The listing builds one solid part. Answer for the finished solid, in the listing's coordinates (mm). Round coordinates to 2 decimals unless told otherwise and drop trailing zeros. Loops run counter-clockwise (first coordinate to the right, second up) from the corner with the lowest first, then second, coordinate; pieces in that order, holes last. Notation, with made-up numbers: (5, 56) - (15, 56) arc R22 cw to (15, 72) - close; hole circle Ø11 at (77, 31.5). An arc over 180 degrees is marked (long way). One line per item, written item: value.
```python
from build123d import *

# Parameters (mm, degrees)
BOSS_EXTRUDE1_DEPTH = 1.7272


with BuildPart() as part:
    # Sketch1 → Boss-Extrude1 (new body)
    with BuildSketch(Plane.XY):
        Polygon((-114.3, 13.37945), (-112.776, 13.37945), (-112.776, 15.10665), (-110.236, 15.10665), (-110.236, 13.37945), (-1.27, 13.37945), (-1.27, 15.10665), (1.27, 15.10665), (1.27, 13.37945), (110.236, 13.37945), (110.236, 15.10665), (112.776, 15.10665), (112.776, 13.37945), (114.3, 13.37945), (114.3, 12.61745), (116.0272, 12.61745), (116.0272, 10.58545), (114.3, 10.58545), (114.3, -7.70255), (116.0272, -7.70255), (116.0272, -9.73455), (114.3, -9.73455), (114.3, -13.37945), (112.776, -13.37945), (112.776, -15.10665), (110.236, -15.10665), (110.236, -13.37945), (1.27, -13.37945), (1.27, -15.10665), (-1.27, -15.10665), (-1.27, -13.37945), (-110.236, -13.37945), (-110.236, -15.10665), (-112.776, -15.10665), (-112.776, -13.37945), (-114.3, -13.37945), (-114.3, -9.73455), (-116.0272, -9.73455), (-116.0272, -7.70255), (-114.3, -7.70255), (-114.3, 10.58545), (-116.0272, 10.58545), (-116.0272, 12.61745), (-114.3, 12.61745), align=None)
        Polygon((-1.27, -1.517324769), (-72.54, -8.677584102), (-72.54, -9.56945), (-1.27, -9.56945), align=None, mode=Mode.SUBTRACT)
        Polygon((-78.89, -6.76276081), (-109.22, -9.80991481), (-109.22, 9.80991481), (-78.89, 6.76276081), align=None, mode=Mode.SUBTRACT)
        Polygon((-11.576521468, 0), (-72.54, -6.124797477), (-72.54, 6.124797477), align=None, mode=Mode.SUBTRACT)
        Polygon((-1.27, 9.56945), (-72.54, 9.56945), (-72.54, 8.677584102), (-1.27, 1.517324769), align=None, mode=Mode.SUBTRACT)
        Polygon((1.27, 1.517324769), (72.54, 8.677584102), (72.54, 9.56945), (1.27, 9.56945), align=None, mode=Mode.SUBTRACT)
        Polygon((78.89, 6.76276081), (109.22, 9.80991481), (109.22, -9.80991481), (78.89, -6.76276081), align=None, mode=Mode.SUBTRACT)
        Polygon((72.54, -6.124797477), (72.54, 6.124797477), (11.576521468, 0), align=None, mode=Mode.SUBTRACT)
        Polygon((1.27, -9.56945), (72.54, -9.56945), (72.54, -8.677584102), (1.27, -1.517324769), align=None, mode=Mode.SUBTRACT)
    extrude(amount=BOSS_EXTRUDE1_DEPTH)


solid = part.part
```
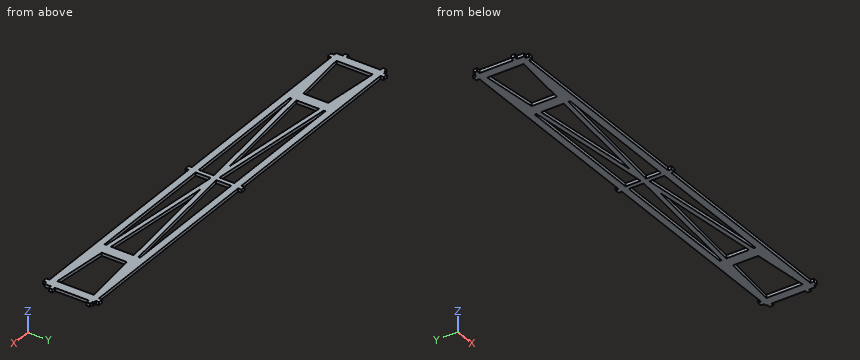
1) A cutting plane is placed at D-D on z = 0.45. Give the number of separate pieces and of enclosed holes in the cut face, and give its area (3 significant figures).
Final values:
separate pieces: 1
enclosed holes: 8
area: 3,130 mm2
2) A cutting plane is placed at C-C on x = -84.5. Give the vertices of the cut face in (y, z).
Final values:
outline: (-13.38, 0) - (-7.33, 0) - (-7.33, 1.73) - (-13.38, 1.73) - close; (7.33, 0) - (13.38, 0) - (13.38, 1.73) - (7.33, 1.73) - close
3) Consider L1, parallel to Y at x = 13.5, z = 0.3; L2, parallel to Y at x = 8, z = 0.25; L3, parallel to Y at x = -53, z = 1.2. Determine where each line is inside the solid, lowest interval first.
Final values:
L1: -13.38 to -9.57, -2.75 to -0.19, 0.19 to 2.75, 9.57 to 13.38
L2: -13.38 to -9.57, -2.19 to 2.19, 9.57 to 13.38
L3: -13.38 to -9.57, -6.71 to -4.16, 4.16 to 6.71, 9.57 to 13.38
4) A cutting plane is placed at A-A on x = -55. Give the vertices of the cut face in (y, z), and give its area (3 significant figures).
Final values:
outline: (-13.38, 0) - (-9.57, 0) - (-9.57, 1.73) - (-13.38, 1.73) - close; (-6.92, 0) - (-4.36, 0) - (-4.36, 1.73) - (-6.92, 1.73) - close; (4.36, 0) - (6.92, 0) - (6.92, 1.73) - (4.36, 1.73) - close; (9.57, 0) - (13.38, 0) - (13.38, 1.73) - (9.57, 1.73) - close
area: 22.0 mm2
5) Each of these flat-tipped pins is pushed along its axis until it touches: pin 1 Ø1 at (y, z) = (9, 1) entering from +X; pin 2 Ø0.5 at (y, z) = (14, 0.5) entering from -X; pin 3 Ø1.5 at (x, y) = (82.5, 5.5) entering from -Z; pin 4 Ø0.5 at (x, z) = (-115, 1) entering from -Y. Where does it stop, or does it pass through?
Final values:
pin 1: x = 114.3
pin 2: x = -112.78
pin 3: through
pin 4: y = -9.73
6) A cutting plane is placed at B-B on y = 4. Give the vertices of the cut face in (x, z).
Final values:
outline: (-114.3, 0) - (-109.22, 0) - (-109.22, 1.73) - (-114.3, 1.73) - close; (-78.89, 0) - (-72.54, 0) - (-72.54, 1.73) - (-78.89, 1.73) - close; (-51.39, 0) - (-25.98, 0) - (-25.98, 1.73) - (-51.39, 1.73) - close; (-1.27, 0) - (1.27, 0) - (1.27, 1.73) - (-1.27, 1.73) - close; (25.98, 0) - (51.39, 0) - (51.39, 1.73) - (25.98, 1.73) - close; (72.54, 0) - (78.89, 0) - (78.89, 1.73) - (72.54, 1.73) - close; (109.22, 0) - (114.3, 0) - (114.3, 1.73) - (109.22, 1.73) - close
